Part model, mm, in its own coordinate system. A direction names the side the tool comes from. Round coordinates to 2 decimals unless told otherwise and drop trailing zeros. Write each loop counter-clockwise with the first axis right and the second up, starting at its lowest first coordinate (ties: lowest second). Pieces come first, ordered by that corner, then holes. Notation, with made-up numbers: (-28.5, 55.25) -> (24.5, 55.25) arc R27 ccw to (24.5, 72.25) -> close; hole circle Ø10 at (60, 21.5). An arc over 180 degrees is marked (long way). Return JSON: item names as keys, results as strings. Group by question number.
(1) Mould opens along Y. For faces 3 (the flat face through (1505, 1543, 501.65)), 4 (the flat face through (1505, 855, 457.2)), 5 (the flat face through (1505, 2057.4, 501)) say: +Y half, -Y half, draft (parallel to the pull), parting line (faces both ways), or undercut.
(2) Saw through at B-B (x = 1504). List the corners of the cut face in (y, z).
(3) Drill centre line: L1, parallel to Y at x = 1495, z = 512. Where is it in solid material? Low to high. Write a range as from..to.
(4) Drop a flat-ended pin along its axis: pin 1 Ø11.5 at (x, y) = (1513, 1542.5) entering from +Z. Give the stop position or say it passes through.
(5) Saw through at A-A (z = 530). List the corners of the cut face in (x, y).
(6) Tool access for faces 1 (the flat face through (1505, 1524, 524)), 2 (the flat face through (1524, 821, 501)): list every direction of +Z, -Z, +X, -X, +Y, -Y with a clear straight run to the whole face (end or side of a thin tool).
from build123d import *

# Parameters (mm, degrees)
BOX007_W        = 38.1
BOX007_H        = 2438.4
BOX007_DEPTH    = 88.9
SKETCH004_W     = 38.1
SKETCH004_H     = 44.45
POCKET004_DEPTH = 38.101


with BuildPart() as pocket004:
    # Box007 → Box007 (new body)
    with BuildSketch(Plane(origin=(0, -381, 457.2), x_dir=(1, 0, 0), z_dir=(0, 0, 1))):
        with Locations((19.05, 1219.2)):
            Rectangle(BOX007_W, BOX007_H)
    extrude(amount=BOX007_DEPTH)

    # Sketch004 → Pocket004 (cut, through all)
    with BuildSketch(Plane(origin=(0, -381, 457.2), x_dir=(0, -1, 0), z_dir=(-1, 0, 0))):
        with Locations((-361.95, 66.675)):
            Rectangle(SKETCH004_W, SKETCH004_H)
        with Locations((-1924.05, 66.675)):
            Rectangle(SKETCH004_W, SKETCH004_H)
    extrude(amount=-POCKET004_DEPTH, mode=Mode.SUBTRACT)


with BuildPart() as eastfloorbeam:
    # Part__Mirroring002: instance of Pocket004
    add(pocket004.part.mirror(Plane(origin=(762, 0, 0), x_dir=(0, -1, 0), z_dir=(1, 0, 0))))


solid = eastfloorbeam.part
Computed values:
{
 "1": {"face 3": "undercut", "face 4": "draft", "face 5": "+Y half"},
 "2": {"outline": "(-381, 457.2) -> (2057.4, 457.2) -> (2057.4, 546.1) -> (1562.1, 546.1) -> (1562.1, 501.65) -> (1524, 501.65) -> (1524, 546.1) -> (0, 546.1) -> (0, 501.65) -> (-38.1, 501.65) -> (-38.1, 546.1) -> (-381, 546.1) -> close"},
 "3": {"L1": "-381..-38.1, 0..1524, 1562.1..2057.4"},
 "4": {"pin 1": "z = 501.65"},
 "5": {"outline": "(1485.9, -381) -> (1524, -381) -> (1524, -38.1) -> (1485.9, -38.1) -> close; (1485.9, 0) -> (1524, 0) -> (1524, 1524) -> (1485.9, 1524) -> close; (1485.9, 1562.1) -> (1524, 1562.1) -> (1524, 2057.4) -> (1485.9, 2057.4) -> close"},
 "6": {"face 1": "+Z, +X, -X", "face 2": "+Z, -Z, +X, +Y, -Y"}
}
